```python
from build123d import *

# Parameters (mm, degrees)
CROQUIS18_R             = 2
CROQUIS18_R_2           = 1.5
CROQUIS18_W             = 20
CROQUIS18_H             = 15
SALIENTE_EXTRUIR1_DEPTH = 3
REDONDEO1_R             = 5


with BuildPart() as part:
    # Croquis18 → Saliente-Extruir1 (new body)
    with BuildSketch(Plane.XY):
        Polygon((-90, -40), (25, -40), (25, -30), (80, -30), (80, -10), (30, -10), (30, 10), (80, 10), (80, 30), (25, 30), (25, 40), (-90, 40), (-90, 20), (-25, 20), (-25, -20), (-90, -20), align=None)
        with Locations((-70.71, -30)):
            Circle(CROQUIS18_R, mode=Mode.SUBTRACT)
        with Locations((-12, -24)):
            Circle(CROQUIS18_R_2, mode=Mode.SUBTRACT)
        with Locations((12, -24)):
            Circle(CROQUIS18_R_2, mode=Mode.SUBTRACT)
        with Locations((70, -20)):
            Circle(CROQUIS18_R, mode=Mode.SUBTRACT)
        with Locations((0, -12.5)):
            Rectangle(CROQUIS18_W, CROQUIS18_H, mode=Mode.SUBTRACT)
        with Locations((-70.71, 30)):
            Circle(CROQUIS18_R, mode=Mode.SUBTRACT)
        with Locations((-12, 24)):
            Circle(CROQUIS18_R_2, mode=Mode.SUBTRACT)
        with Locations((0, 12.5)):
            Rectangle(CROQUIS18_W, CROQUIS18_H, mode=Mode.SUBTRACT)
        with Locations((70, 20)):
            Circle(CROQUIS18_R, mode=Mode.SUBTRACT)
        with Locations((12, 24)):
            Circle(CROQUIS18_R_2, mode=Mode.SUBTRACT)
    extrude(amount=SALIENTE_EXTRUIR1_DEPTH)

    # Redondeo1
    redondeo1_edges = [part.edges().sort_by_distance(p)[0] for p in [
        (25, -40, 1.5),
        (25, -30, 1.5),
        (25, 40, 1.5),
        (25, 30, 1.5),
        (-25, -20, 1.5),
        (-25, 20, 1.5),
        (-90, -40, 1.5),
        (-90, -20, 1.5),
        (-90, 20, 1.5),
        (-90, 40, 1.5),
        (80, 30, 1.5),
        (80, -30, 1.5),
        (30, -10, 1.5),
        (30, 10, 1.5),
        (80, -10, 1.5),
        (80, 10, 1.5),
    ]]
    fillet(redondeo1_edges, radius=REDONDEO1_R - 0.0001)  # a hair under: the kernel refuses the full size


solid = part.part
```
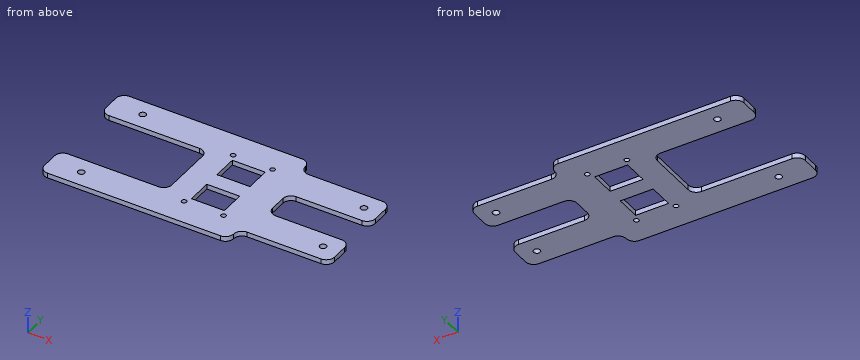
CAD build for the part. Positions are in the model's coordinates, mm. Coordinates: 2 decimals unless noted, no trailing zeros. Order: outer loops, then holes, each group sorted by start corner. A loop starts at its lowest first (then second) coordinate and runs counter-clockwise, first axis right, second up. Notation, with made-up numbers: M 3.25,-32 L 29.25,-32 A24 ccw 29.25,-10 Z; hole C 4,-7.75 d2. An arc over 180 degrees is marked long. Write each question's results on one line, items separated by ' | '. Start each with the question number.
Q1. Cut at D-D (z = 2.55). Count the separate pieces of the cut face and the enclosed holes in it, then the cut area to 3 significant figures.
Q2. Cut at C-C (x = 4). List the corners of the cut face in (y, z).
Q3. Flat gauge pins, fed straight in: P1, Ø1.5, axis at y = -15, z = 1.5, coming from the -X side; P2, Ø1.5, axis at y = -8.5, z = 2, coming from the +X side; P3, Ø1.5, axis at y = 2, z = 1, coming from the -X side. Where does each tip first touch, or does it go through?
Q4. Cut at A-A (x = -40). List the corners of the cut face in (y, z).
Q5. Drill centre lines: probe 1 along Y at (x, z) = (12, 1.55); probe 2 along Y at (x, z) = (-70.71, 1.5); probe 3 along Y at (x, z) = (37, 1.75). Where is each one in solid material? Low to high. Write a range as from..to.
Q6. Cut at B-B (x = -70.71). List the corners of the cut face in (y, z).
Found:
1) separate pieces: 1 | enclosed holes: 10 | area: 8,200 mm²
2) outline: M -40,0 L -20,0 L -20,3 L -40,3 Z; M -5,0 L 5,0 L 5,3 L -5,3 Z; M 20,0 L 40,0 L 40,3 L 20,3 Z
3) P1: x = -25.06 | P2: x = 32.37 | P3: x = -25
4) outline: M -40,0 L -20,0 L -20,3 L -40,3 Z; M 20,0 L 40,0 L 40,3 L 20,3 Z
5) probe 1: -40..-25.5, -22.5..22.5, 25.5..40 | probe 2: -40..-32, -28..-20, 20..28, 32..40 | probe 3: -30..-10, 10..30
6) outline: M -40,0 L -32,0 L -32,3 L -40,3 Z; M -28,0 L -20,0 L -20,3 L -28,3 Z; M 20,0 L 28,0 L 28,3 L 20,3 Z; M 32,0 L 40,0 L 40,3 L 32,3 Z
